Input: part model. Units: mm. Frame: model coordinates. A direction names the side the tool comes from. Round coordinates to 2 decimals unless told otherwise and drop trailing zeros. Loops run counter-clockwise (first coordinate to the right, second up) from the corner with the lowest first, then second, coordinate; pieces in that order, holes last. Notation, with made-up numbers: M 46.25,6.25 L 77.25,6.25 A13 cw 77.25,28.25 Z; hole C -7.75,-16 d9. An arc over 180 degrees is marked long. Put each result on its own line as item: value. Start each with the question number.
1) Line query: probe 1 along Z at (x, y) = (0, 8.5); probe 2 along X at (y, z) = (-3.79, 26.85) (3 decimals); probe 3 along Z at (x, y) = (11.5, 30). Output: solid intervals per line, ascending.
2) Section A-A on y = 0. Output: boundary loops of the cut face in (x, z) (3 decimals).
3) Section C-C on y = 13. Output: boundary loops of the cut face in (x, z).
4) Pin query (flat end, axial travel): pin 1 (6 mm diameter, centred on x = -25.5, y = 25, fed in from +Z); pin 2 (10 mm diameter, centred on x = 6, y = 27, fed in from +Z); pin 3 (3.5 mm diameter, centred on x = 0, z = 26.5, fed in from -Y). Return the tip coordinate at first contact, or that it passes through.
5) Section B-B on x = 0. State how many separate pieces and enclosed holes the cut face has, plus the area to 3 significant figures.
6) Reachability of faces 1 (the face through (0, 37.15, 27)), 2 (the face through (0, 33.65, 26)), 3 (the face through (-3.545, 0, 27)) from +Z, -Z, +X, -X, +Y, -Y: full face, straight path, thin tool, end or side. Return the list, or none.
7) Section D-D on x = -20.5. Output: boundary loops of the cut face in (y, z), plus the area to 3 significant figures.
8) Draft query along X for faces 4 (the face through (3.545, 0, 27)), 5 (the face through (0.65, -2.22, 27.25)), 6 (the face through (0, -32.15, 21)). Return one class per face: +X half, -X half, draft (parallel to the pull), parting line (faces both ways), or undercut.
from build123d import *

# Parameters (mm, degrees)
SKETCH004_R             = 37.65
PAD002_DEPTH            = 2
SKETCH005_R             = 2.75
SKETCH005_R_2           = 1.75
PAD003_DEPTH            = 32.65
SKETCH007_R             = 4.05
PAD004_DEPTH            = 5
POCKET_DEPTH            = 4
PAD014_DEPTH            = 4
SKETCH006_R             = 1.75
POCKET003012_DEPTH      = 75.219717
SKETCH036_R             = 1.7
POCKET003013_DEPTH      = 5
BODY001_PLACEMENT_ANGLE = 90


with BuildPart() as part:
    # Sketch004 → Pad002 (new body)
    with BuildSketch(Plane.XY):
        Circle(SKETCH004_R)
    extrude(amount=PAD002_DEPTH)

    # Sketch005 → Pad003 (join, symmetric)
    with BuildSketch(Plane(origin=(0, 0, 1), x_dir=(0, 1, 0), z_dir=(1, 0, 0))):
        Circle(SKETCH005_R)
        Circle(SKETCH005_R_2, mode=Mode.SUBTRACT)
    extrude(amount=PAD003_DEPTH, both=True)

    # Sketch007 → Pad004 (join)
    with BuildSketch(Plane(origin=(37.15, 0, 1), x_dir=(0, 1, 0), z_dir=(1, 0, 0))):
        Circle(SKETCH007_R)
    pad004 = extrude(amount=-PAD004_DEPTH)

    # Mirrored: Pad004 across YZ
    add(pad004.mirror(Plane.YZ))

    # Sketch008 → Pocket (cut)
    with BuildSketch(Plane(origin=(37.65, 0, 1), x_dir=(0, 1, 0), z_dir=(1, 0, 0))):
        Polygon((1.525, -2.641377), (3.05, 0), (1.525, 2.641377), (-1.525, 2.641377), (-3.05, 0), (-1.525, -2.641377), align=None)
    pocket = extrude(amount=-POCKET_DEPTH, mode=Mode.SUBTRACT)

    # Mirrored001: Pocket across YZ
    add(pocket.mirror(Plane.YZ), mode=Mode.SUBTRACT)

    # Sketch035 → Pad014 (join)
    with BuildSketch(Plane.XY.offset(6)):
        with BuildLine():
            ThreePointArc((-4.82, 3.545), (-8.365, 0), (-4.82, -3.545))
            Line((-4.82, -3.545), (4.82, -3.545))
            ThreePointArc((4.82, -3.545), (8.365, 0), (4.82, 3.545))
            Line((4.82, 3.545), (-4.82, 3.545))
        make_face()
    extrude(amount=-PAD014_DEPTH)

    # Sketch006 → Pocket003012 (cut, through all)
    with BuildSketch(Plane(origin=(37.65, 0, 1), x_dir=(0, 1, 0), z_dir=(1, 0, 0))):
        Circle(SKETCH006_R)
    extrude(amount=-POCKET003012_DEPTH, mode=Mode.SUBTRACT)

    # Sketch036 → Pocket003013 (cut)
    with BuildSketch(Plane.XY.offset(6)):
        with Locations((-3.79, 0)):
            Circle(SKETCH036_R)
    pocket003013 = extrude(amount=-POCKET003013_DEPTH, mode=Mode.SUBTRACT)

    # Mirrored002: Pocket003013 across Sketch036 V_Axis
    add(pocket003013.mirror(Plane(origin=(0, 0, 6), x_dir=(0, 0, 1), z_dir=(1, 0, 0))), mode=Mode.SUBTRACT)


with BuildPart() as part_1:
    # Body001 placement: moved
    add(part.part.moved(Location((0, 0, 23))).rotate(Axis((0, 0, 23), (0, 0, 1)), BODY001_PLACEMENT_ANGLE))


solid = part_1.part
Geometry results:
1. probe 1: z = 21.25 to 22.25, 25.75 to 26.75
1. probe 2: x = -3.545 to -1.7, 1.7 to 3.545
1. probe 3: z = 23 to 25
2. outline: M -37.65,23 L -2.562,23 A2.75 ccw 2.562,23 L 37.65,23 L 37.65,25 L 3.545,25 L 3.545,29 L -3.545,29 L -3.545,25 L -37.65,25 Z; hole C 0,24 d3.5
3. outline: M -35.33,23 L -2.56,23 A2.75 ccw 2.56,23 L 35.33,23 L 35.33,25 L 2.56,25 A2.75 ccw -2.56,25 L -35.33,25 Z; hole C 0,24 d3.5
4. pin 1: stops at z = 25
4. pin 2: stops at z = 26.56
4. pin 3: stops at y = -37.15
5. separate pieces: 4
5. enclosed holes: 0
5. area: 178 mm²
6. face 1: +Z, +X, -X, +Y
6. face 2: +Y
6. face 3: +Z, -X
7. outline: M -31.58,23 L 31.58,23 L 31.58,25 L -31.58,25 Z
7. area: 126 mm²
8. face 4: +X half
8. face 5: undercut
8. face 6: draft
